from build123d import *

# Parameters (mm, degrees)
F0_R          = 10
F1_DEPTH      = 42.5
F3_D          = 8.5
F3_DEPTH      = 20
F3_TIP        = 2.5536576309
F4_SIZE       = 1
F5_W          = 50
F5_H          = 7
F6_DEPTH      = 10.001
F6_DEPTH_BACK = 10.001
F7_R          = 2


with BuildPart() as f1:
    # F0 (on Front) → F1 (new body, symmetric)
    with BuildSketch(Plane.XZ):
        Circle(F0_R)
    extrude(amount=F1_DEPTH, both=True)

    # F3
    with Locations(Plane.XZ.offset(42.5)):
        with Locations((0, 0)):
            Hole(F3_D / 2, depth=F3_DEPTH)
            with Locations((0, 0, -(F3_DEPTH + F3_TIP / 2))):  # 118° drill point
                Cone(0, F3_D / 2, F3_TIP, mode=Mode.SUBTRACT)

    # F4
    f4_edges = [f1.edges().sort_by_distance(p)[0] for p in [
        (-10, 42.5, 0),
    ]]
    chamfer(f4_edges, length=F4_SIZE)

    # F5 (on Right) → F6 (cut, two sides)
    with BuildSketch(Plane.YZ) as f6_sk:
        with Locations((7.5, 6.5)):
            Rectangle(F5_W, F5_H)
    extrude(amount=-F6_DEPTH, mode=Mode.SUBTRACT)
    extrude(f6_sk.sketch, amount=F6_DEPTH_BACK, mode=Mode.SUBTRACT)

    # F7
    f7_edges = [f1.edges().sort_by_distance(p)[0] for p in [
        (0, -17.5, 3),
        (0, 32.5, 3),
    ]]
    fillet(f7_edges, radius=F7_R)


solid = f1.part
Work out the finished part from the listing and answer in its coordinate system (mm). A direction names the side the tool comes from. Round coordinates to 2 decimals unless told otherwise and drop trailing zeros. Write each loop counter-clockwise with the first axis right and the second up, starting at its lowest first coordinate (ties: lowest second). Pieces come first, ordered by that corner, then holes. Notation, with made-up numbers: (35.5, -13) - (59.5, -13) arc R30 ccw to (59.5, 24) - close; hole circle Ø5 at (-16.75, 64.5). An arc over 180 degrees is marked (long way). Answer in a Markdown table with one row per item. Add a question column.
1. Find the intervals of material crossed by line 1 along Z through (x, y) = (0, -30); line 2 along Y through (x, z) = (-6, 5.5); line 3 along X through (y, z) = (-4, -5), in increasing order. Write a range as from..to.
2. Given pin 1 (7.5 mm diameter, centred on x = 0, z = 0, fed in from -Y); pin 2 (10 mm diameter, centred on y = 13, z = -5.5, fed in from +X); pin 3 (5.5 mm diameter, centred on x = 2.5, y = 11, fed in from +Z), each flat-ended and moving along its own axis, determine where each tip first touches the part or whether it passes through.
3. For faces 4 (the cylindrical face through (-0.13, 31.93, 3.6)), 5 (the flat face through (0, 42.5, 0)), determine the directions among +Z, -Z, +X, -X, +Y, -Y from which every point of the face is accessible in a straight line to the end or side of a thin tool.
4. A cutting plane is placed at A-A, the plane y = -21. Determine the outline of the cut face in (x, z).
5. The mould has two halves that part along Y. Classify faces 1 (the flat face through (2, -42.5, -4)), 2 (the flat face through (0, 32.5, 7)), 3 (the cylindrical face through (-2.285, -32.36, 3.584)): +Y half, -Y half, draft (parallel to the pull), parting line (faces both ways), or undercut.
Worked out:
| question | item | result |
|---|---|---|
| 1 | line 1 | -10..-4.25, 4.25..10 |
| 1 | line 2 | -42.5..-17.5, 32.5..42.5 |
| 1 | line 3 | -8.66..8.66 |
| 2 | pin 1 | y = -22.2 |
| 2 | pin 2 | x = 9.99 |
| 2 | pin 3 | z = 3 |
| 3 | face 4 | +Z, +X, -X |
| 3 | face 5 | +Z, -Z, +X, -X, +Y |
| 4 | outline | circle Ø20 at (0, 0); hole circle Ø3.51 at (0, 0) |
| 5 | face 1 | -Y half |
| 5 | face 2 | undercut |
| 5 | face 3 | draft |
